Autodesk Inventor part; units mm, degrees
ref_plane "Arbeitsebene1" through (0, 0, 3.8) normal (0, 0, 1) x (1, 0, 0)
ref_plane "Arbeitsebene2" through (0, 0, 0) normal (1, 0, 0) x (0, 1, 0)
ref_plane "Arbeitsebene3" through (0, 0, 2.4) normal (0, 0, -1) x (-1, 0, 0)
sketch "Skizze3" plane through (0, 0, 0) normal (0, 0, 1) x (1, 0, 0)
  circle A0 centre (0, 0) radius 1.25
  dimension "d0" = 2.5
extrude "Extrusion1" add sketch "Skizze3" along normal blind 4.8
ref_plane "Arbeitsebene1" through (0, 0, 3.8) normal (0, 0, 1) x (1, 0, 0)
split_face "Trennen1"
ref_plane "Arbeitsebene2" through (0, 0, 0) normal (1, 0, 0) x (0, 1, 0)
sketch "Skizze6" plane through (0, 0, 0) normal (1, 0, 0) x (0, 1, 0)
  line L0 (0, 4.8) -> (0, 8.5)
  arc A0 (0, 8.5) -> (-0.25, 8.75) centre (-0.25, 8.5) ccw
  line L1 (-0.25, 8.5) -> (-0.25, 8.75) construction
  line L2 (-0.25, 8.5) -> (0, 8.5) construction
  line L3 (-0.25, 8.75) -> (-4.25, 8.75)
  line L4 (1.25, 4.8) -> (-1.25, 4.8)
  line L5 (1.25, 4.8) -> (1.25, 3.8)
  line L6 (1.25, 3.8) -> (1.25, 0)
  line L7 (1.25, 0) -> (-1.25, 0)
  line L8 (-1.25, 0) -> (-1.25, 3.8)
  line L9 (-1.25, 3.8) -> (-1.25, 4.8)
  line L10 (-1.25, 4.8) -> (1.25, 4.8)
  line L11 (-1.25, 3.8) -> (-1.25, 4.8)
  point P0 (0, 0)
  dimension "d7" = 90
  dimension "d9" = 3.7
  dimension "d10" = 4
  dimension "d13" = 0.25
  dimension "d20" = 0.25
  dimension "d21" = 1.25
sketch "Skizze4" plane through (0, 0, 4.8) normal (0, 0, 1) x (1, 0, 0)
  circle A0 centre (0, 0) radius 0.25
  dimension "d4" = 0.5
sweep "Sweeping1" add profiles "Skizze4" path "Skizze6" path curves L0 A0 L3
ref_plane "Arbeitsebene3" through (0, 0, 2.4) normal (0, 0, -1) x (-1, 0, 0)
mirror "Spiegeln1" about plane through (0, 0, 2.4) normal (0, 0, -1) of "Sweeping1"
properties part number "Diode"
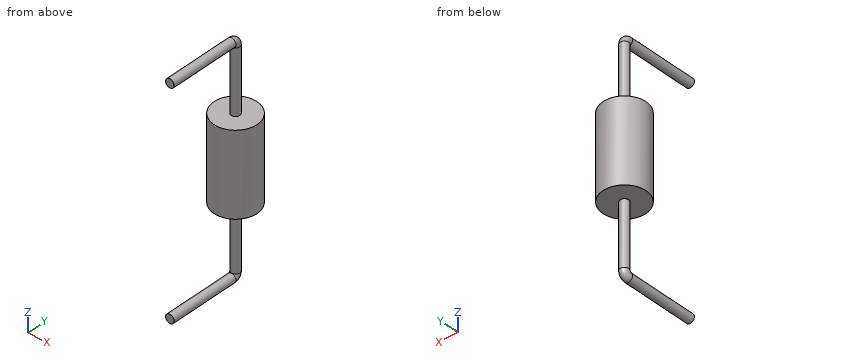
Model file for the job. Use its own axes, mm. Round coordinates to 2 decimals unless told otherwise and drop trailing zeros. Write each loop counter-clockwise with the first axis right and the second up, starting at its lowest first coordinate (ties: lowest second). Pieces come first, ordered by that corner, then holes. Notation, with made-up numbers: (22, 88) - (66, 88) arc R12 ccw to (66, 105) - close; hole circle Ø1 at (-23.75, 29). An arc over 180 degrees is marked (long way). Use CSV: the item, a comma, the result in double quotes. Start each with the question number.
Item 1: Band-saw the part on D-D (x = -0.8). Write the cut outline in (y, z), and give its area (3 significant figures).
Item 2: Band-saw the part on C-C (z = 3.75). Write the cut outline in (x, y).
Item 3: Drill centre lines: L1, parallel to Z at x = -0.05, y = -3.5; L2, parallel to Z at x = -0.15, y = -2.2; L3, parallel to Y at x = -0.05, z = 7. Where is each one in solid material? Low to high. Write a range as [from, to].
Item 4: Pin check, flat tip, straight feed: P1, Ø1.5, axis at x = 0.5, z = 6, coming from the -Y side. Stop position of the tip, or through.
Item 5: Band-saw the part on A-A (y = -3.3). Write the cut outline in (x, z).
Checked values:
1,outline,"(-0.96, 0) - (0.96, 0) - (0.96, 4.8) - (-0.96, 4.8) - close"
1,area,"9.22 mm²"
2,outline,"circle Ø2.5 at (0, 0)"
3,L1,"z = [-4.19, -3.71], [8.51, 8.99]"
3,L2,"z = [-4.15, -3.75], [8.55, 8.95]"
3,L3,"y = [-0.24, 0.24]"
4,P1,"stops at y = -0.25"
5,outline,"circle Ø0.5 at (0, -3.95); circle Ø0.5 at (0, 8.75)"
